Geometry check sheet. Reference: drawing and pictorial views, mm from the part's lowest x, y, z. A direction names the side the tool comes from. Round coordinates to 2 decimals unless told otherwise and drop trailing zeros. Write each loop counter-clockwise with the first axis right and the second up, starting at its lowest first coordinate (ties: lowest second). Pieces come first, ordered by that corner, then holes. Notation, with made-up numbers: M 23.5,-38 L 44.5,-38 A38 ccw 44.5,1 Z; hole C 41.5,9.25 d3. An arc over 180 degrees is marked long. Put each result on its own line as item: value. Start each with the question number.
(1) Gauge pin test, flat ends, axial feed: pin 1 (3 mm diameter, centred on x = 13.5, y = 15.5, fed in from +Z); pin 2 (4.5 mm diameter, centred on x = 15, y = 26, fed in from -Z); pin 3 (1.5 mm diameter, centred on y = 22, z = 1.5, fed in from +X); pin 4 (2.5 mm diameter, centred on x = 4, y = 15, fed in from +Z). Record the tip position at first contact, or that the pin passes through.
(2) Section check C-C on z = 2.35. Record the cut outline in (x, y).
(3) Material ranges on probe 1 along Y at (x, z) = (15, 1.45); probe 2 along Y at (x, z) = (15, 2.3); probe 3 along X at (y, z) = (15.5, 1.25), recorded low to high.
(4) Mould release check, pull along X, two halves, no side actions. Record for the marked faces 4, 5 and 6: pulls with the +X half, pulls with the -X half, needs draft (parallel to the pull), parting line crosses it, or undercut.
(5) Section check D-D on y = 26.75. Record the cut outline in (x, z).
(6) Tool access check on the marked faces 1, 2 and 3. Record the directions out of +Z, -Z, +X, -X, +Y, -Y that give a thin tool (end or side, any length) a straight path to the whole face; none if there is none.
(7) Section check A-A on x = 15. Record the cut outline in (y, z), then the cut area to 3 significant figures.
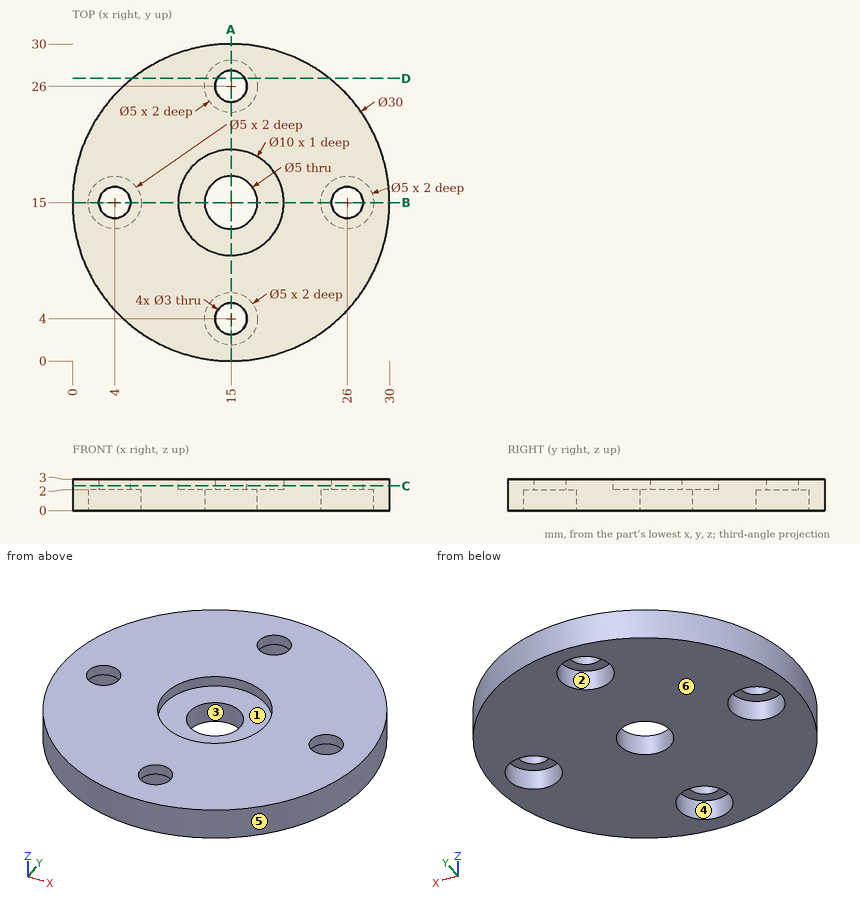
Answers follow:
1. pin 1: stops at z = 2
1. pin 2: stops at z = 2
1. pin 3: stops at x = 28.64
1. pin 4: passes through
2. outline: C 15,15 d30; hole C 4,15 d3; hole C 15,15 d10; hole C 15,4 d3; hole C 15,26 d3; hole C 26,15 d3
3. probe 1: y = 0 to 1.5, 6.5 to 12.5, 17.5 to 23.5, 28.5 to 30
3. probe 2: y = 0 to 2.5, 5.5 to 10, 20 to 24.5, 27.5 to 30
3. probe 3: x = 0.01 to 1.55, 6.45 to 12.55, 17.45 to 23.55, 28.45 to 29.99
4. face 4: undercut
4. face 5: parting line crosses it
4. face 6: needs draft
5. outline: M 5.68,0 L 12.62,0 L 12.62,2 L 13.7,2 L 13.7,3 L 5.68,3 Z; M 16.3,2 L 17.38,2 L 17.38,0 L 24.32,0 L 24.32,3 L 16.3,3 Z
6. face 1: +Z
6. face 2: -Z
6. face 3: +Z, -Z
7. outline: M 0,0 L 1.5,0 L 1.5,2 L 2.5,2 L 2.5,3 L 0,3 Z; M 5.5,2 L 6.5,2 L 6.5,0 L 12.5,0 L 12.5,2 L 10,2 L 10,3 L 5.5,3 Z; M 17.5,0 L 23.5,0 L 23.5,2 L 24.5,2 L 24.5,3 L 20,3 L 20,2 L 17.5,2 Z; M 27.5,2 L 28.5,2 L 28.5,0 L 30,0 L 30,3 L 27.5,3 Z
7. area: 44.0 mm^2
